For this review, take the finished solid that the model builds, in its own axes (mm). A direction names the side the tool comes from. Round coordinates to 2 decimals unless told otherwise and drop trailing zeros. Loops run counter-clockwise (first coordinate to the right, second up) from the corner with the lowest first, then second, coordinate; pieces in that order, holes last.
1. Consider section B-B on x = 0. State how many separate pieces and enclosed holes the cut face has, then the cut area to 3 significant figures.
2. Tool access review of faces 4 (the cylindrical face through (9.39, -21.65, 4.93)), 5 (the flat face through (16.8, 3, 39)), 6 (the flat face through (2.25, -20, 3)), 7 (the flat face through (15.8, 11, 5)), 8 (the flat face through (4.8, 0, 6)): name each direction out of +Z, -Z, +X, -X, +Y, -Y from which nothing blocks a thin tool from reaching the whole face with its end or side.
3. Clearance check with flat-ended pins moving along their axes: pin 1 Ø2 at (y, z) = (0.5, 32) entering from +X; pin 2 Ø12 at (y, z) = (-8.5, 9) entering from -X; pin 3 Ø3.5 at (y, z) = (0, 6.2) entering from -X; pin 4 Ø2.5 at (x, z) = (-12.5, 63.5) entering from +Y. State where each tip first meets the part, or that it passes through.
4. Consider section A-A on z = 31.5. State the section outline as (x, y) points.
5. Draft analysis for pull direction X (two halves, no side actions). For faces 1 (the flat face through (15.8, -11, 5)), 2 (the cylindrical face through (12.55, -2.46, 14)), 3 (the conical face through (0.988, 23.104, -3.812)), state which applies: released by +X, released by -X, zero draft, split by the parting line, or undercut.
6. To check wall thickness, follow line 1 along X through (y, z) = (-1.5, 31.5); line 2 along X through (y, z) = (-3, 47); line 3 along X through (y, z) = (1, 52). State the ranges of each line that lie inside material, in increasing order.
Autodesk Fusion 360 part; units mm, degrees
sketch "Schizzo1" plane through (0, 0, 0) normal (0, 0, 1) x (1, 0, 0)
  circle A0 centre (0, 0) radius 25
  line L0 (0, 0) -> (0, 25) construction
  line L1 (0, 0) -> (0, -25) construction
  line L2 (-15.8, 19.3742) -> (-15.8, 17.5305) construction
  line L3 (-15.8, 17.5305) -> (-15.8, -17.5305)
  line L4 (-15.8, -17.5305) -> (-15.8, -19.3742) construction
  line L5 (15.8, 19.3742) -> (15.8, 17.5305) construction
  line L6 (15.8, 17.5305) -> (15.8, -17.5305)
  line L7 (15.8, -17.5305) -> (15.8, -19.3742) construction
  arc A1 (15.8, 17.5305) -> (-15.8, 17.5305) centre (0, 0) ccw
  arc A2 (-15.8, -17.5305) -> (15.8, -17.5305) centre (0, 0) ccw
  line L8 (-15.8, 0) -> (-19.8, 0) construction
  line L9 (15.8, 0) -> (19.8, 0) construction
  line L10 (-19.8, 0) -> (-19.8, 5)
  line L11 (-19.8, 5) -> (-15.8, 5)
  line L12 (-19.8, 0) -> (-19.8, -5)
  line L13 (-19.8, -5) -> (-15.8, -5)
  line L14 (19.8, 0) -> (19.8, 5)
  line L15 (19.8, 5) -> (15.8, 5)
  line L16 (19.8, 0) -> (19.8, -5)
  line L17 (19.8, -5) -> (15.8, -5)
  circle A3 centre (0, 0) radius 2
  circle A4 centre (0, -16) radius 2.75
  circle A5 centre (0, 10) radius 2
  line L18 (13.723, 19.2) -> (-13.723, 19.2)
  line L19 (2.25, -17.5811) -> (2.25, -24.8985)
  line L20 (-2.25, -17.5811) -> (-2.25, -24.8985)
  dimension "d1" = 50
  dimension "d3" = 31.6
  dimension "d4" = 1.4
  dimension "d5" = 10
  dimension "d6" = 4
  dimension "d21" = 4
  dimension "d22" = 5.5
  dimension "d23" = 16
  dimension "d39" = 4
  dimension "d40" = 10
  dimension "d45" = 5.8
  dimension "d48" = 4.5
extrude "Estrusione1" add sketch "Schizzo1" along normal blind 10 contours L3 L6 A1 A2 A4 L18 L19 L20 | L3 L10 L11 L12 L13 | L6 L14 L15 L16 L17
extrude "Estrusione2" add sketch "Schizzo1" against normal blind 4 contours A0 L3 L6 A1 A2 L10 L11 L12 L13 L14 L15 L16 L17 L19 L20 | L3 L6 A1 A2 A4 L18 L19 L20 | L3 L10 L11 L12 L13 | L6 L14 L15 L16 L17 | A1 L18
sketch "Schizzo2" plane through (-19.8, 0, 0) normal (-1, 0, 0) x (0, -1, 0)
  line L0 (-5, 0) -> (5, 0)
  line L1 (5, 0) -> (5, 10)
  line L2 (5, 10) -> (-5, 10)
  line L3 (-5, 10) -> (-5, 0)
  line L4 (0, 0) -> (0, 6.2) construction
  circle A0 centre (0, 6.2) radius 2
  dimension "d11" = 6.2
  dimension "d12" = 4
extrude "Estrusione3" cut sketch "Schizzo2" against normal blind 15 contours A0
sketch "Schizzo3" plane through (19.8, 0, 0) normal (1, 0, 0) x (0, 1, 0)
  line L0 (-5, 0) -> (5, 0)
  line L1 (5, 0) -> (5, 10)
  line L2 (5, 10) -> (-5, 10)
  line L3 (-5, 10) -> (-5, 0)
  circle A0 centre (0, 6.2) radius 2
  circle A1 centre (0, 6.2) radius 2
extrude "Estrusione4" cut sketch "Schizzo3" against normal blind 15 contours A0 A1
chamfer "Smusso1" distance 1 angle 45 2 edges at (0, -13.25, -4) (-1.8647, -0.7232, -4)
chamfer "Smusso3" distance 2 distance2 3 1 edges at (0, 25, -4) measured on face at (-8.7268, -9.7213, -4)
fillet "Raccordo1" radius 2 1 edges at (-1.8647, -0.7232, -3)
sketch "Schizzo7" plane through (0, 0, 10) normal (0, 0, 1) x (-1, 0, 0)
  circle A0 centre (0, 0) radius 2
  circle A1 centre (0, -10) radius 2
  line L0 (-2.25, 17.5811) -> (-2.25, 23.4925)
  arc A2 (-2.25, 23.4925) -> (-15.8, 17.5305) centre (0, 0) ccw
  line L1 (-15.8, 17.5305) -> (-15.8, 5)
  line L2 (-15.8, 5) -> (-19.8, 5)
  line L3 (-19.8, 5) -> (-19.8, -5)
  line L4 (-19.8, -5) -> (-15.8, -5)
  line L5 (-15.8, -5) -> (-15.8, -17.5305)
  arc A3 (-15.8, -17.5305) -> (-13.723, -19.2) centre (0, 0) ccw
  line L6 (-13.723, -19.2) -> (13.723, -19.2)
  arc A4 (13.723, -19.2) -> (15.8, -17.5305) centre (0, 0) ccw
  line L7 (15.8, -17.5305) -> (15.8, -5)
  line L8 (15.8, -5) -> (19.8, -5)
  line L9 (19.8, -5) -> (19.8, 5)
  line L10 (19.8, 5) -> (15.8, 5)
  line L11 (15.8, 5) -> (15.8, 17.5305)
  arc A5 (15.8, 17.5305) -> (2.25, 23.4925) centre (0, 0) ccw
  line L12 (2.25, 23.4925) -> (2.25, 17.5811)
  arc A6 (-2.25, 17.5811) -> (2.25, 17.5811) centre (0, 16) ccw
  line L13 (15.8, -5) -> (16.8, -5)
  line L14 (16.8, -5) -> (16.8, 0)
  line L15 (16.8, 0) -> (10, 0)
  line L16 (10, 0) -> (10, 5)
  line L17 (10, 5) -> (15.8, 5)
  line L18 (-15.8, -5) -> (-16.8, -5)
  line L19 (-16.8, -5) -> (-16.8, 0)
  line L20 (-16.8, 0) -> (-10, 0)
  line L21 (-10, 0) -> (-10, 5)
  line L22 (-10, 5) -> (-15.8, 5)
  dimension "d49" = 3
  dimension "d50" = 20
  dimension "d51" = 5
extrude "Estrusione6" add sketch "Schizzo7" along normal blind 59 contours L2 L3 L4 L19 L20 L21 L22 | L8 L9 L10 L14 L15 L16 L17
sketch "Schizzo8" plane through (0, 0, 69) normal (0, 0, 1) x (-1, 0, 0)
  line L0 (16.8, -5) -> (19.8, -5)
  line L1 (19.8, -5) -> (19.8, 5)
  line L2 (19.8, 5) -> (10, 5)
  line L3 (10, 5) -> (10, 0)
  line L4 (10, 0) -> (16.8, 0)
  line L5 (16.8, 0) -> (16.8, -5)
  line L6 (-10, 5) -> (-19.8, 5)
  line L7 (-19.8, 5) -> (-19.8, -5)
  line L8 (-19.8, -5) -> (-16.8, -5)
  line L9 (-16.8, -5) -> (-16.8, 0)
  line L10 (-16.8, 0) -> (-10, 0)
  line L11 (-10, 0) -> (-10, 5)
  line L12 (-10, 5) -> (10, 5)
  line L13 (-10, 0) -> (10, 0)
extrude "Estrusione7" add sketch "Schizzo8" against normal blind 10 contours L3 L11 L12 L13
sketch "Schizzo9" plane through (0, 0, 0) normal (0, 1, 0) x (-1, 0, 0)
  line L0 (10, 10) -> (16.8, 10)
  line L1 (16.8, 10) -> (16.8, 69)
  line L2 (16.8, 69) -> (-16.8, 69)
  line L3 (-16.8, 69) -> (-16.8, 10)
  line L4 (-16.8, 10) -> (-10, 10)
  line L5 (-10, 10) -> (-10, 59)
  line L6 (-10, 59) -> (10, 59)
  line L7 (10, 59) -> (10, 10)
  line L8 (-12.5, 69) -> (-12.5, 10) construction
  line L9 (0, 69) -> (0, 59) construction
  line L10 (-13.4642, 40.6491) -> (-12.5, 41.4581)
  line L11 (-12.5, 41.4581) -> (-11.5358, 40.6491)
  arc A0 (-13.4642, 40.6491) -> (-11.5358, 40.6491) centre (-12.5, 39.5) ccw
  arc A1 (-13.4642, 16.6491) -> (-11.5358, 16.6491) centre (-12.5, 15.5) ccw
  line L12 (-12.5, 17.4581) -> (-11.5358, 16.6491)
  line L13 (-13.4642, 16.6491) -> (-12.5, 17.4581)
  arc A2 (11.5358, 16.6491) -> (13.4642, 16.6491) centre (12.5, 15.5) ccw
  line L14 (12.5, 17.4581) -> (13.4642, 16.6491)
  line L15 (11.5358, 16.6491) -> (12.5, 17.4581)
  arc A3 (-13.4642, 24.6491) -> (-11.5358, 24.6491) centre (-12.5, 23.5) ccw
  line L16 (-12.5, 25.4581) -> (-11.5358, 24.6491)
  line L17 (-13.4642, 24.6491) -> (-12.5, 25.4581)
  arc A4 (11.5358, 24.6491) -> (13.4642, 24.6491) centre (12.5, 23.5) ccw
  line L18 (12.5, 25.4581) -> (13.4642, 24.6491)
  line L19 (11.5358, 24.6491) -> (12.5, 25.4581)
  arc A5 (-13.4642, 32.6491) -> (-11.5358, 32.6491) centre (-12.5, 31.5) ccw
  line L20 (-12.5, 33.4581) -> (-11.5358, 32.6491)
  line L21 (-13.4642, 32.6491) -> (-12.5, 33.4581)
  arc A6 (11.5358, 32.6491) -> (13.4642, 32.6491) centre (12.5, 31.5) ccw
  line L22 (12.5, 33.4581) -> (13.4642, 32.6491)
  line L23 (11.5358, 32.6491) -> (12.5, 33.4581)
  arc A7 (11.5358, 40.6491) -> (13.4642, 40.6491) centre (12.5, 39.5) ccw
  line L24 (12.5, 41.4581) -> (13.4642, 40.6491)
  line L25 (11.5358, 40.6491) -> (12.5, 41.4581)
  arc A8 (-13.4642, 48.6491) -> (-11.5358, 48.6491) centre (-12.5, 47.5) ccw
  line L26 (-12.5, 49.4581) -> (-11.5358, 48.6491)
  line L27 (-13.4642, 48.6491) -> (-12.5, 49.4581)
  arc A9 (11.5358, 48.6491) -> (13.4642, 48.6491) centre (12.5, 47.5) ccw
  line L28 (12.5, 49.4581) -> (13.4642, 48.6491)
  line L29 (11.5358, 48.6491) -> (12.5, 49.4581)
  arc A10 (-13.4642, 56.6491) -> (-11.5358, 56.6491) centre (-12.5, 55.5) ccw
  line L30 (-12.5, 57.4581) -> (-11.5358, 56.6491)
  line L31 (-13.4642, 56.6491) -> (-12.5, 57.4581)
  arc A11 (11.5358, 56.6491) -> (13.4642, 56.6491) centre (12.5, 55.5) ccw
  line L32 (12.5, 57.4581) -> (13.4642, 56.6491)
  line L33 (11.5358, 56.6491) -> (12.5, 57.4581)
  arc A12 (-13.4642, 64.6491) -> (-11.5358, 64.6491) centre (-12.5, 63.5) ccw
  line L34 (-12.5, 65.4581) -> (-11.5358, 64.6491)
  line L35 (-13.4642, 64.6491) -> (-12.5, 65.4581)
  arc A13 (11.5358, 64.6491) -> (13.4642, 64.6491) centre (12.5, 63.5) ccw
  line L36 (12.5, 65.4581) -> (13.4642, 64.6491)
  line L37 (11.5358, 64.6491) -> (12.5, 65.4581)
  dimension "d57" = 12.5
  dimension "d58" = 50
  dimension "d59" = 1.5
  dimension "d62" = 25
  dimension "d63" = 8
extrude "Estrusione8" cut sketch "Schizzo9" against normal blind 5 contours L10 L11 A0 | A1 L12 L13 | A2 L14 L15 | A3 L16 L17 | A4 L18 L19 | A5 L20 L21 | A6 L22 L23 | A7 L24 L25 | A8 L26 L27 | A9 L28 L29 | A10 L30 L31 | A11 L32 L33 | A12 L34 L35 | A13 L36 L37
fillet "Raccordo5" radius 1 4 edges at (19.8, -5, 34.5) (19.8, 5, 34.5) (-19.8, -5, 34.5) (-19.8, 5, 34.5)
fillet "Raccordo6" radius 1 6 edges at (15.8, -17.5305, 5) (13.723, 19.2, 5) (15.8, 17.5305, 5) (-15.8, 17.5305, 5) (-13.723, 19.2, 5) (-15.8, -17.5305, 5)
component "Component" placed x (1, 0, 0) y (0, 1, 0) z (0, 0, 1) at (0, 0, 0)
Resolved:
1. separate pieces: 4
1. enclosed holes: 0
1. area: 411 mm2
2. face 4: +Z, +X, -Y
2. face 5: +Z, +Y
2. face 6: +Z, -Z, -Y
2. face 7: +Z, +X, +Y
2. face 8: +X
3. pin 1: stops at x = 19.8
3. pin 2: stops at x = -19.8
3. pin 3: stops at x = -4.8
3. pin 4: passes through
4. outline: (-19.8, -4) arc R1 ccw to (-18.8, -5) - (-14, -5) - (-14, 0) - (-16.8, 0) - (-16.8, 5) - (-18.8, 5) arc R1 ccw to (-19.8, 4) - close; (-11, -5) - (-10, -5) - (-10, 0) - (-11, 0) - close; (10, -5) - (11, -5) - (11, 0) - (10, 0) - close; (14, -5) - (18.8, -5) arc R1 ccw to (19.8, -4) - (19.8, 4) arc R1 ccw to (18.8, 5) - (16.8, 5) - (16.8, 0) - (14, 0) - close
5. face 1: released by +X
5. face 2: undercut
5. face 3: split by the parting line
6. line 1: x = -19.8 to -14, -11 to -10, 10 to 11, 14 to 19.8
6. line 2: x = -19.8 to -13.91, -11.09 to -10, 10 to 11.09, 13.91 to 19.8
6. line 3: x = -19.8 to -16.8, 16.8 to 19.8
